The listing builds one solid part. Answer for the finished solid, in the listing's coordinates (mm). Give positions to 0.01 mm unless a question says otherwise; leave off trailing zeros. Answer in a Markdown table with one row per item. Add a question column.
from build123d import *

# Parameters (mm, degrees)
F0_W     = 139.7
F0_H     = 38.1
F1_DEPTH = 203.2
F2_R     = 6.35
F3_SIZE  = 6.35
F4_SIZE  = 6.35
F5_R     = 6.35
F6_DEPTH = 2.54


with BuildPart() as f1:
    # F0 (on Front) → F1 (new body)
    with BuildSketch(Plane.XZ):
        Rectangle(F0_W, F0_H)
    extrude(amount=F1_DEPTH)

    # F2
    f2_edges = [f1.edges().sort_by_distance(p)[0] for p in [
        (-69.85, -101.6, 19.05),
        (-69.85, -101.6, -19.05),
        (69.85, -101.6, 19.05),
        (69.85, -101.6, -19.05),
    ]]
    fillet(f2_edges, radius=F2_R)

    # F3
    f3_edges = [f1.edges().sort_by_distance(p)[0] for p in [
        (0, -203.2, 19.05),
    ]]
    chamfer(f3_edges, length=F3_SIZE)

    # F4
    f4_edges = [f1.edges().sort_by_distance(p)[0] for p in [
        (0, 0, 19.05),
    ]]
    chamfer(f4_edges, length=F4_SIZE)

    # F5 (on face) → F6 (cut)
    with BuildSketch(Plane(origin=(0, 0, 0), x_dir=(-1, 0, 0), z_dir=(0, 1, 0))):
        with Locations((50.8, 0)):
            Circle(F5_R)
    extrude(amount=-F6_DEPTH, mode=Mode.SUBTRACT)


solid = f1.part
1. The mould has two halves that part along X. Classify faces 1 (the face through (-56.857, -1.252, 1.907)), 2 (the face through (66.7, -200, 0.2)), 3 (the face through (-1, -100, 19.05)): +X half, -X half, draft (parallel to the pull), parting line (faces both ways), or undercut.
2. Given pin 1 Ø7.5 at (x, z) = (-50.8, 0) entering from +Y, flat-ended and moving along its own axis, determine where the tip first touches the part or whether it passes through.
3. Straight lines are drawn through the part: L1, parallel to Z at x = -50.8, y = -0.6; L2, parallel to Z at x = -50.8, y = -1.5; L3, parallel to Y at x = -12, z = -14. For each, find the intervals that lie inside material, in ascending order. Write a range as [from, to].
Geometry check:
| question | item | result |
|---|---|---|
| 1 | face 1 | undercut |
| 1 | face 2 | +X half |
| 1 | face 3 | draft |
| 2 | pin 1 | y = -2.54 |
| 3 | L1 | [-13.3, -6.35], [6.35, 13.3] |
| 3 | L2 | [-14.2, -6.35], [6.35, 14.2] |
| 3 | L3 | [-201.9, -1.3] |
